from build123d import *

# Parameters (mm, degrees)
F0_R     = 154.8
F0_R_2   = 4
F0_R_3   = 85
F1_DEPTH = 25.4


with BuildPart() as f1:
    # F0 (on Front) → F1 (new body)
    with BuildSketch(Plane.XZ):
        Circle(F0_R)
        with Locations((-90.350369, -29.356614)):
            Circle(F0_R_2, mode=Mode.SUBTRACT)
        with Locations((-55.839599, -76.856614)):
            Circle(F0_R_2, mode=Mode.SUBTRACT)
        with Locations((0, -95)):
            Circle(F0_R_2, mode=Mode.SUBTRACT)
        with Locations((55.839599, -76.856614)):
            Circle(F0_R_2, mode=Mode.SUBTRACT)
        with Locations((90.350369, -29.356614)):
            Circle(F0_R_2, mode=Mode.SUBTRACT)
        with Locations((-90.350369, 29.356614)):
            Circle(F0_R_2, mode=Mode.SUBTRACT)
        with Locations((-55.839599, 76.856614)):
            Circle(F0_R_2, mode=Mode.SUBTRACT)
        Circle(F0_R_3, mode=Mode.SUBTRACT)
        with Locations((55.839599, 76.856614)):
            Circle(F0_R_2, mode=Mode.SUBTRACT)
        with Locations((90.350369, 29.356614)):
            Circle(F0_R_2, mode=Mode.SUBTRACT)
        with Locations((0, 95)):
            Circle(F0_R_2, mode=Mode.SUBTRACT)
    extrude(amount=F1_DEPTH)


solid = f1.part
Here's how the part is built. I have some questions about the finished solid (model axes, mm). Round coordinates to 2 decimals unless told otherwise and drop trailing zeros. Loops run counter-clockwise (first coordinate to the right, second up) from the corner with the lowest first, then second, coordinate; pieces in that order, holes last. Notation, with made-up numbers: M 20,-6 L 44,-6 A12 cw 44,8 Z; hole C 55,-37.75 d7. An arc over 180 degrees is marked long. Write each question's results on one line, items separated by ' | '. Start each with the question number.
(1) I want a section at A-A (x = 0). Please give me the cut outline in (y, z), then the cut area to 3 significant figures.
(2) I want a section at D-D (y = -19.5). State how many separate pieces and enclosed holes the cut face has, then the cut area to 3 significant figures.
(3) I want a section at C-C (x = 68). Please give me the cut outline in (y, z).
(4) If I drill on probe 1 along Z at (x, y) = (0, -15.5); probe 2 along Z at (x, y) = (88.5, -4.25); probe 3 along Z at (x, y) = (55, -19), over which ranges is the centre line in solid material (lowest first)? Write a range as from..to.
(5) Will these pins go through, and if not, where does the flat tip stop? P1, Ø3, axis at x = -118.5, z = -27.5, coming from the +Y side; P2, Ø4, axis at x = -17.5, y = -17.5, coming from the +Z side; P3, Ø7, axis at x = 0, z = 95, coming from the -Y side; P4, Ø2, axis at x = -120.5, y = -15, coming from the +Z side.
(6) I want a section at B-B (z = 0). Please give me the cut outline in (x, y).
(7) Thinking about a two-plate mould opening in X: for faces 1 (the flat face through (67, -25.4, -67)), 2 (the cylindrical face through (-154.65, -12.52, 6.81)), 3 (the cylindrical face through (55.319, -12.522, 80.823)), 4 (the cylindrical face through (-52.024, -12.522, -75.655)), which applies, pulls with the +X half, pulls with the -X half, needs draft (parallel to the pull), parting line crosses it, or undercut?
Solved:
1) outline: M -25.4,-154.8 L 0,-154.8 L 0,-99 L -25.4,-99 Z; M -25.4,-91 L 0,-91 L 0,-85 L -25.4,-85 Z; M -25.4,85 L 0,85 L 0,91 L -25.4,91 Z; M -25.4,99 L 0,99 L 0,154.8 L -25.4,154.8 Z | area: 3,140 mm²
2) separate pieces: 1 | enclosed holes: 11 | area: 52,100 mm²
3) outline: M -25.4,-139.06 L 0,-139.06 L 0,-51 L -25.4,-51 Z; M -25.4,51 L 0,51 L 0,139.06 L -25.4,139.06 Z
4) probe 1: z = -154.8..-99, -91..-85, 85..91, 99..154.8 | probe 2: z = -127.01..-32.9, -25.81..25.81, 32.9..127.01 | probe 3: z = -144.7..-80.77, -72.95..-64.81, 64.81..72.95, 80.77..144.7
5) P1: stops at y = 0 | P2: stops at z = 154.02 | P3: passes through | P4: stops at z = 98.4
6) outline: M -154.8,-25.4 L -85,-25.4 L -85,0 L -154.8,0 Z; M 85,-25.4 L 154.8,-25.4 L 154.8,0 L 85,0 Z
7) face 1: needs draft | face 2: parting line crosses it | face 3: undercut | face 4: undercut
